```python
from build123d import *

# Parameters (mm, degrees)
BOSS_EXTRUDE1_DEPTH = 6
SKETCH5_W           = 50.780974492
SKETCH5_H           = 22.085020173
SKETCH5_R           = 5
CUT_EXTRUDE1_DEPTH  = 1
CHAMFER2_SIZE       = 0.5


with BuildPart() as part:
    # Sketch2 → Boss-Extrude1 (new body)
    with BuildSketch(Plane(origin=(0, 0, 0), x_dir=(1, 0, 0), z_dir=(0, 1, 0))):
        with BuildLine():
            Line((0, 5), (23, 5))
            ThreePointArc((23, 5), (28, 0), (23, -5))
            Line((23, -5), (0, -5))
            ThreePointArc((0, -5), (-5, 0), (0, 5))
        make_face()
    extrude(amount=BOSS_EXTRUDE1_DEPTH)

    # Sketch3 → Cut-Revolve1 (revolve, cut)
    with BuildSketch(Plane.XY):
        Polygon((0, 0), (-3.75, 0), (-3.75, 3.5), (-2.075, 3.5), (-2.075, 6), (0, 6), align=None)
    revolve(axis=Axis((0, 0, 0), (0, 1, 0)), mode=Mode.SUBTRACT)

    # Sketch4 → Cut-Revolve2 (revolve, cut)
    with BuildSketch(Plane.XY):
        Polygon((23, 0), (19.25, 0), (19.25, 3.5), (20.925, 3.5), (20.925, 6), (23, 6), align=None)
    revolve(axis=Axis((23, 0, 0), (0, 1, 0)), mode=Mode.SUBTRACT)

    # Sketch5 → Cut-Extrude1 (cut)
    with BuildSketch(Plane(origin=(0, 6, 0), x_dir=(1, 0, 0), z_dir=(0, 1, 0))):
        with Locations((10.314830551, 0.079491573)):
            Rectangle(SKETCH5_W, SKETCH5_H)
        Circle(SKETCH5_R, mode=Mode.SUBTRACT)
        with Locations((23, 0)):
            Circle(SKETCH5_R, mode=Mode.SUBTRACT)
    extrude(amount=-CUT_EXTRUDE1_DEPTH, mode=Mode.SUBTRACT)

    # Chamfer2
    chamfer2_edges = [part.edges().sort_by_distance(p)[0] for p in [
        (23, 6, 5),
        (2.075, 6, 0),
        (25.075, 6, 0),
        (-5, 6, 0),
        (11.5, 0, -5),
        (28, 0, 0),
        (11.5, 0, 5),
        (-5, 0, 0),
    ]]
    chamfer(chamfer2_edges, length=CHAMFER2_SIZE)


solid = part.part
```
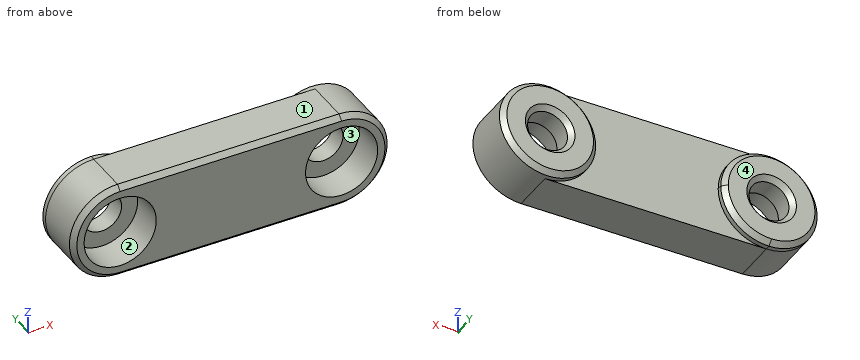
Build history of the part. All positions in model axes, mm. Face numbers are marked on the shaded views. A direction names the side the tool comes from. Round coordinates to 2 decimals unless told otherwise and drop trailing zeros. Loops run counter-clockwise (first coordinate to the right, second up) from the corner with the lowest first, then second, coordinate; pieces in that order, holes last.
Item 1: Saw through at A-A (y = 2.9). List the corners of the cut face in (x, z).
Item 2: Saw through at B-B (x = 16.5). List the corners of the cut face in (y, z).
Item 3: Which spindle directions (+Z, -Z, +X, -X, +Y, -Y) get a long thin tool onto all of the face, cutting with end or side? Do the marked faces 1 and 2. Say none if no direction does.
Item 4: Two-plate mould, pull along X, no slides. Class the marked faces 3 and 4: released by +X, released by -X, zero draft, split by the parting line, or undercut.
Item 5: Pin check, flat tips, straight feed: P1, Ø6, axis at x = 23, z = 0, coming from the -Y side; P2, Ø5, axis at x = 23, z = 0, coming from the +Y side (3 decimals); P3, Ø3, axis at x = 11, z = 0, coming from the +Y side. Stop position of each tip, or through.
Item 6: Saw through at C-C (z = 1.5). State how many separate pieces and enclosed holes the cut face has, then the cut area to 3 significant figures.
Item 7: Drill centre lines: line 1 along Z through (x, y) = (0, 4.35) (3 decimals); line 2 along Z through (x, y) = (0, 2.7); line 3 along X through (y, z) = (1.75, 1). Where is each one in solid material? Low to high.
Worked answers:
1. outline: (0, -5) - (23, -5) arc R5 ccw to (23, 5) - (0, 5) arc R5 ccw to start; hole circle Ø7.5 at (0, 0); hole circle Ø7.5 at (23, 0)
2. outline: (0, -4.5) - (0.5, -5) - (5, -5) - (5, 5) - (0.5, 5) - (0, 4.5) - close
3. face 1: +Z, +X, -X, +Y, -Y
3. face 2: -Y
4. face 3: undercut
4. face 4: zero draft
5. P1: stops at y = 3.5
5. P2: stops at y = 5.925
5. P3: stops at y = 5
6. separate pieces: 3
6. enclosed holes: 0
6. area: 118 mm2
7. line 1: z = -5 to -2.075, 2.075 to 5
7. line 2: z = -5 to -3.75, 3.75 to 5
7. line 3: x = -4.9 to -3.61, 3.61 to 19.39, 26.61 to 27.9
